The listing builds one solid part. Answer for the finished solid, in the listing's coordinates (mm). Face numbers are marked on the shaded views. A direction names the side the tool comes from. Round coordinates to 2 decimals unless told otherwise and drop trailing zeros. Write each loop counter-clockwise with the first axis right and the second up, starting at its lowest first coordinate (ties: lowest second). Pieces come first, ordered by that corner, then holes. Notation, with made-up numbers: (65.5, 61) - (101.5, 61) arc R23 ccw to (101.5, 74) - close; hole circle Ø6 at (80, 13.25). An arc over 180 degrees is marked (long way). Return JSON: item names as keys, results as strings. Group by question number.
(1) Find the intervals of material crossed by line 1 along Y through (x, z) = (0, 0.5); line 2 along Z through (x, y) = (5.25, 1); line 3 along Y through (x, z) = (0, -8.75), in increasing order. Write a range as [from, to].
(2) Each of these flat-tipped pins is pushed along its axis until it touches: pin 1 (5 mm diameter, centred on x = -7, z = -3, fed in from -Y); pin 2 (10 mm diameter, centred on y = -5.5, z = 6.5, fed in from -X); pin 3 (1 mm diameter, centred on x = -8, z = 6.5, fed in from -Y). Where does it stop, or does it pass through?
(3) Section D-D, the plane x = -4 is taken. Write down the section's boundary in (y, z), then the cut area to 3 significant figures.
(4) Which of the six approach directions +Z, -Z, +X, -X, +Y, -Y give full straight-line access (tool end or side, diameter ignored) to the marked faces 4, 5 and 6?
(5) Section A-A, the plane y = 0 is taken. Write down the section's boundary in (x, z) (3 decimals).
(6) Determine the mould class of the marked faces 1, 2 and 3 for opening direction Y: +Y half, -Y half, draft (parallel to the pull), parting line (faces both ways), or undercut.
(7) Section C-C, the plane z = 9 is taken. Write down the section's boundary in (x, y) (3 decimals), then the cut area to 3 significant figures.
(8) Section B-B, the plane x = 0 is taken. Write down the section's boundary in (y, z), then the cut area to 3 significant figures.
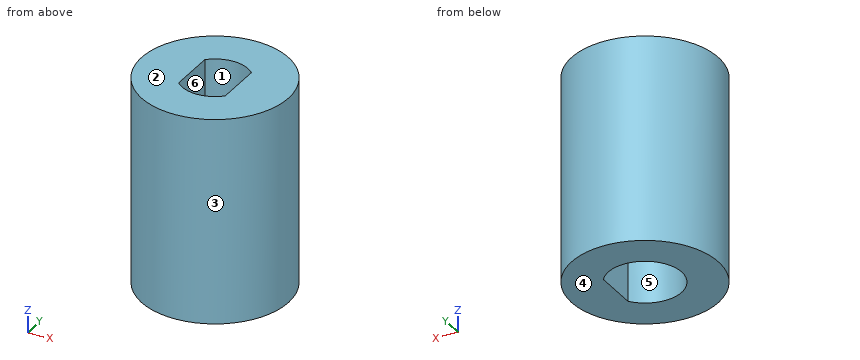
```python
from build123d import *

# Parameters (mm, degrees)
SKETCH_1_R          = 10
EXTRUDE_1_DEPTH     = 14
SKETCH_3_R          = 6
CUT_EXTRUDE_1_DEPTH = 5
SKETCH_2_R          = 4.5
EXTRUDE_2_DEPTH     = 9


with BuildPart() as part:
    # 草图1 → 凸台-拉伸1 (new, symmetric)
    with BuildSketch(Plane.XY):
        Circle(SKETCH_1_R)
        with BuildLine():
            Line((4, 3), (4, -3))
            ThreePointArc((4, -3), (-5, 0), (4, 3))
        make_face(mode=Mode.SUBTRACT)
    extrude(amount=EXTRUDE_1_DEPTH, both=True)

    # 草图3 → 切除-拉伸1 (cut, symmetric)
    with BuildSketch(Plane.XY):
        Circle(SKETCH_3_R)
    extrude(amount=CUT_EXTRUDE_1_DEPTH, both=True, mode=Mode.SUBTRACT)

    # 草图2 → 凸台-拉伸2 (add)
    # profile 1 of 4: a face of its own
    with BuildSketch(Plane.XY.offset(14)):
        with BuildLine():
            Line((4, 3), (4, -3))
            ThreePointArc((4, -3), (-5, 0), (4, 3))
        make_face()
        Circle(SKETCH_2_R, mode=Mode.SUBTRACT)
    # profile 2 of 4: a face of its own
    with BuildSketch(Plane.XY.offset(14)):
        with BuildLine():
            ThreePointArc((-3.175, 3.188945751), (-4.5, 0), (-3.175, -3.188945751))
            Line((-3.175, -3.188945751), (-3.175, 3.188945751))
        make_face()
    # profile 3 of 4: a face of its own
    with BuildSketch(Plane.XY.offset(14)):
        with BuildLine():
            Line((4, 2.061552813), (4, -2.061552813))
            ThreePointArc((4, -2.061552813), (4.373213921, -1.060660172), (4.5, 0))
            ThreePointArc((4.5, 0), (4.373213921, 1.060660172), (4, 2.061552813))
        make_face()
    # profile 4 of 4: a face of its own
    with BuildSketch(Plane.XY.offset(14)):
        with BuildLine():
            ThreePointArc((3.175, -3.188945751), (3.631516207, -2.657459321), (4, -2.061552813))
            Line((4, -2.061552813), (4, 2.061552813))
            ThreePointArc((4, 2.061552813), (3.631516207, 2.657459321), (3.175, 3.188945751))
            Line((3.175, 3.188945751), (3.175, -3.188945751))
        make_face()
    extrude(amount=-EXTRUDE_2_DEPTH)


solid = part.part
```
Working result:
{
 "1": {"line 1": "y = [-10, -6], [6, 10]", "line 2": "z = [-14, -5], [5, 14]", "line 3": "y = [-10, -5], [5, 10]"},
 "2": {"pin 1": "stops at y = -8.93", "pin 2": "stops at x = -9.99", "pin 3": "stops at y = -6.61"},
 "3": {"outline": "(-9.17, -14) - (-3, -14) - (-3, -5) - (-4.47, -5) - (-4.47, 5) - (4.47, 5) - (4.47, -5) - (3, -5) - (3, -14) - (9.17, -14) - (9.17, 14) - (-9.17, 14) - close", "area": "370 mm^2"},
 "4": {"face 4": "-Z, +X, -X, +Y, -Y", "face 5": "-Z", "face 6": "+Z, -Z"},
 "5": {"outline": "(-10, -14) - (-5, -14) - (-5, -5) - (-6, -5) - (-6, 5) - (-3.175, 5) - (-3.175, 14) - (-10, 14) - close; (3.175, 5) - (6, 5) - (6, -5) - (4, -5) - (4, -14) - (10, -14) - (10, 14) - (3.175, 14) - close"},
 "6": {"face 1": "undercut", "face 2": "draft", "face 3": "parting line"},
 "7": {"outline": "circle Ø20 at (0, 0); hole (-3.175, -3.189) arc R4.5 ccw to (3.175, -3.189) - (3.175, 3.189) arc R4.5 ccw to (-3.175, 3.189) - close", "area": "262 mm^2"},
 "8": {"outline": "(-10, -14) - (-5, -14) - (-5, -5) - (-6, -5) - (-6, 5) - (-4.5, 5) - (-4.5, 14) - (-10, 14) - close; (4.5, 5) - (6, 5) - (6, -5) - (5, -5) - (5, -14) - (10, -14) - (10, 14) - (4.5, 14) - close", "area": "269 mm^2"}
}
